Autodesk Fusion 360 part; units mm, degrees
sketch "Sketch1" plane through (0, 0, 0) normal (0, 1, 0) x (1, 0, 0)
  line L0 (8.4, 0) -> (15.75, 0)
  line L1 (15.75, 0) -> (15.85, -7.5)
  line L2 (15.85, -7.5) -> (18.5, -7.5)
  line L3 (18.5, -7.5) -> (18.5, -8.8)
  line L4 (18.5, -8.8) -> (15, -9.8)
  line L5 (15, -9.8) -> (0, -9.8)
  line L6 (0, -9.8) -> (0, -0.35)
  line L7 (8.4, 0) -> (8.4, -0.35)
  line L8 (8.4, -0.35) -> (0, -0.35)
  dimension "d2" = 15.85
  dimension "d3" = 15.75
  dimension "d4" = 7.5
  dimension "d5" = 18.5
  dimension "d6" = 9.8
  dimension "d7" = 15
  dimension "d8" = 1.3
  dimension "d9" = 0.35
  dimension "d10" = 8.4
revolve "Revolve1" add sketch "Sketch1" angle 360 about axis through (0, 0, 9.8) along (0, 0, -1)
equation "d2 = ( 31.7 / 2 ) * 1 mm"
equation "d3 = ( 31.5 / 2 ) * 1 mm"
equation "d5 = ( 37 / 2 ) * 1 mm"
equation "d10 = ( 16.8 / 2 ) * 1 mm"
Source: CAD feature listing. Evaluate the final solid. Frame: model axes, mm. A direction names the side the tool comes from. Give positions to 0.01 mm unless a question says otherwise; leave off trailing zeros. Write each loop counter-clockwise with the first axis right and the second up, starting at its lowest first coordinate (ties: lowest second). Pieces come first, ordered by that corner, then holes. Notation, with made-up numbers: M -30.75,89.5 L 11.25,89.5 A21 cw 11.25,120.5 Z; hole C 14,28.25 d8. An arc over 180 degrees is marked long. Answer as a JSON object with one key per item and string values.
Q1. Access query for faces 1 (the face through (0, 0, 9.8)), 2 (the face through (-3.425, -15.425, 3.803)). Directions: +Z, -Z, +X, -X, +Y, -Y. A direction counts if a zero-diameter tool reaches every point of the face in a straight line with its end or side. Return the directions, or none.
Geometry check:
{"face 1": "+Z, +X, -X, +Y, -Y", "face 2": "-Z"}
Q2. Cut plane B-B, the plane z = 2.75. Return the cut outline in (x, y).
Geometry check:
{"outline": "C 0,0 d31.57"}
Q3. Mould query, pull axis X, two halves, no side actions, for faces 3 (the face through (-3.299, 14.857, 9.737)), 4 (the face through (8.012, 2.523, 0.177)), 5 (the face through (7, 7, 0)). Classes: +X half, -X half, draft (parallel to the pull), parting line (faces both ways), or undercut.
Geometry check:
{"face 3": "parting line", "face 4": "undercut", "face 5": "draft"}
Q4. Ray query, line 1 along Y through (x, z) = (0, 0.1). Return the intervals inside material, ascending.
Geometry check:
{"line 1": "y = -15.75 to -8.4, 8.4 to 15.75"}
Q5. Contact query for flat-ended pins moving along their axis: P1, Ø2, axis at y = 13, z = 2.5, coming from the -X side; P2, Ø1.5, axis at x = 13, y = -13, coming from the +Z side; P3, Ø1.5, axis at x = -3, z = 6.5, coming from the +Y side. Output: stop coordinate, or through.
Geometry check:
{"P1": "stops at x = -10.25", "P2": "stops at z = 9.05", "P3": "stops at y = 15.68"}
Q6. Cut plane A-A, the plane z = 4.75. Return the cut outline in (x, y), then the cut area to 3 significant figures.
Geometry check:
{"outline": "C 0,0 d31.63", "area": "786 mm^2"}
